For this review, take the finished solid that the model builds, in its own axes (mm). Face numbers are marked on the shaded views. A direction names the side the tool comes from. Coordinates: 2 decimals unless noted, no trailing zeros. Loops run counter-clockwise (first coordinate to the right, second up) from the corner with the lowest first, then second, coordinate; pieces in that order, holes last. Notation, with made-up numbers: (68, -8.5) -> (77, -8.5) arc R20 ccw to (77, 20.5) -> close; hole circle Ø2 at (80, 37.5). An arc over 180 degrees is marked (long way). Answer in a Markdown table with one row per item.
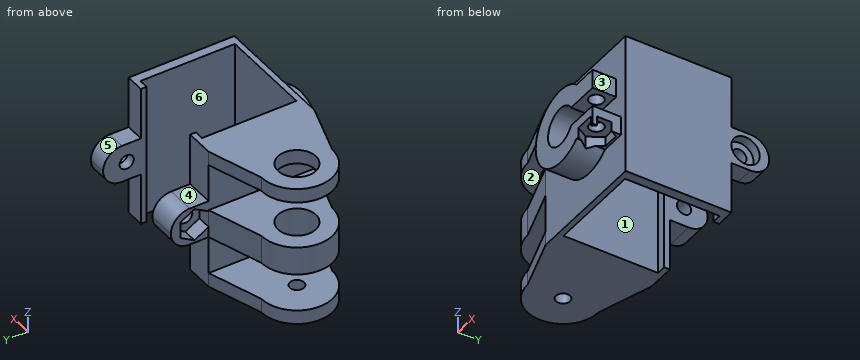
from build123d import *

# Parameters (mm, degrees)
F1_DEPTH  = 30
F3_DEPTH  = 6
F4_DEPTH  = 25
F6_DEPTH  = 15
F7_R      = 1.5
F8_DEPTH  = 25
F9_W      = 4
F9_H      = 8
F9_W_2    = 6
F10_DEPTH = 8
F11_R     = 3.99999
F12_R     = 1.5
F13_DEPTH = 25
F14_START = 27
F0_R      = 1.5
F14_DEPTH = 3
F15_START = 11
F15_DEPTH = 6
F16_DEPTH = 3
F17_R     = 4
F17_R_2   = 1.5
F18_DEPTH = 27
F12_R_2   = 3
F19_DEPTH = 2
F21_DEPTH = 3
F23_START = -2
F22_R     = 1.5
F23_DEPTH = 8


# Not quite as in the source:
# - a fillet or chamfer is up to 0.001 mm smaller than in the source, because OpenCascade refuses the exact size
# - a feature names something its author has since deleted; it is built from what else it names


with BuildPart() as f1:
    # F0 (on Top) → F1 (new body)
    with BuildSketch(Plane.XY):
        Polygon((20, 0), (0, 0), (0, 20), (2, 20), (2, 21.2), (-4, 21.2), (-4, -1.2), (22, -1.2), (22, 21.2), (18, 21.2), (18, 20), (20, 20), align=None)
    extrude(amount=F1_DEPTH)

    # F2 (on face) → F3 (join)
    with BuildSketch(Plane.XZ.offset(1.2)):
        with BuildLine():
            ThreePointArc((6, 15), (8.9647238196, 18.8637033052), (13.4641016151, 17))
            Line((13.4641016151, 17), (17.7459666924, 17))
            ThreePointArc((17.7459666924, 17), (16.8186436725, 19.1840289755), (15.2915026221, 21))
            ThreePointArc((15.2915026221, 21), (6.7084973779, 22.2915026221), (2, 15))
            Line((2, 15), (6, 15))
        make_face()
        with BuildLine():
            ThreePointArc((15.2915026221, 21), (16.8186436725, 19.1840289755), (17.7459666924, 17))
            Line((17.7459666924, 17), (20.4641016151, 17))
            Line((20.4641016151, 17), (20.4641016151, 21))
            Line((20.4641016151, 21), (15.2915026221, 21))
        make_face()
        with BuildLine():
            Line((20.4641016151, 13), (17.7459666924, 13))
            ThreePointArc((17.7459666924, 13), (16.8186436725, 10.8159710245), (15.2915026221, 9))
            Line((15.2915026221, 9), (20.4641016151, 9))
            Line((20.4641016151, 9), (20.4641016151, 13))
        make_face()
        with BuildLine():
            Line((17.7459666924, 13), (13.4641016151, 13))
            ThreePointArc((13.4641016151, 13), (8.9647238196, 11.1362966948), (6, 15))
            Line((6, 15), (2, 15))
            ThreePointArc((2, 15), (6.7084973779, 7.7084973779), (15.2915026221, 9))
            ThreePointArc((15.2915026221, 9), (16.8186436725, 10.8159710245), (17.7459666924, 13))
        make_face()
    extrude(amount=F3_DEPTH)

    # F2 (on face) → F4 (cut)
    with BuildSketch(Plane.XZ.offset(1.2)):
        with BuildLine():
            ThreePointArc((13.4641016151, 13), (13.8637033052, 13.9647238196), (14, 15))
            ThreePointArc((14, 15), (13.8637033052, 16.0352761804), (13.4641016151, 17))
            ThreePointArc((13.4641016151, 17), (8.9647238196, 18.8637033052), (6, 15))
            ThreePointArc((6, 15), (8.9647238196, 11.1362966948), (13.4641016151, 13))
        make_face()
    extrude(amount=-F4_DEPTH, mode=Mode.SUBTRACT)

    # F5 (on face) → F6 (cut)
    with BuildSketch(Plane.XY.offset(30)):
        Polygon((22, -1.2), (3, -1.2), (3, -2.2), (23, -2.2), (23, -1.2), align=None)
    extrude(amount=-F6_DEPTH, mode=Mode.SUBTRACT)

    # F7 (on face) → F8 (cut)
    with BuildSketch(Plane.XY.offset(21)):
        with Locations((17.8778021186, -4.7)):
            Circle(F7_R)
    extrude(amount=-F8_DEPTH, mode=Mode.SUBTRACT)

    # F9 (on face) → F10 (join)
    with BuildSketch(Plane(origin=(0, 21.2, 0), x_dir=(-1, 0, 0), z_dir=(0, 1, 0))):
        with Locations((-20, 15)):
            Rectangle(F9_W, F9_H)
        with Locations((1, 15)):
            Rectangle(F9_W_2, F9_H)
    extrude(amount=F10_DEPTH)

    # F11 (radius 4 in the source; OpenCascade refuses exactly that, so slightly less here)
    f11_edges = [f1.edges().sort_by_distance(p)[0] for p in [
        (20, 29.2, 19),
        (20, 29.2, 11),
        (-1, 29.2, 19),
        (-1, 29.2, 11),
    ]]
    fillet(f11_edges, radius=F11_R)

    # F12 (on face) → F13 (cut)
    with BuildSketch(Plane.YZ.offset(22)):
        with Locations((24.2, 15)):
            Circle(F12_R)
    extrude(amount=-F13_DEPTH, mode=Mode.SUBTRACT)

    # F0 (on Top) → F14 (join)
    with BuildSketch(Plane.XY.offset(F14_START)):
        with BuildLine():
            Line((-4, -1.2), (-4, 21.2))
            Line((-4, 21.2), (-15.5, 17.5))
            ThreePointArc((-15.5, 17.5), (-10.1966991411, 15.3033008589), (-8, 10))
            ThreePointArc((-8, 10), (-10.1966991411, 4.6966991411), (-15.5, 2.5))
            Line((-15.5, 2.5), (-4, -1.2))
        make_face()
        with BuildLine():
            ThreePointArc((-8, 10), (-10.1966991411, 15.3033008589), (-15.5, 17.5))
            ThreePointArc((-15.5, 17.5), (-23, 10), (-15.5, 2.5))
            ThreePointArc((-15.5, 2.5), (-10.1966991411, 4.6966991411), (-8, 10))
        make_face()
        with Locations((-15.5, 10)):
            Circle(F0_R, mode=Mode.SUBTRACT)
        Polygon((20, 0), (0, 0), (0, 20), (2, 20), (2, 21.2), (-4, 21.2), (-4, -1.2), (22, -1.2), (22, 21.2), (18, 21.2), (18, 20), (20, 20), align=None)
    extrude(amount=F14_DEPTH)

    # F0 (on Top) → F15 (join)
    with BuildSketch(Plane.XY.offset(F15_START)):
        with BuildLine():
            ThreePointArc((-8, 10), (-10.1966991411, 15.3033008589), (-15.5, 17.5))
            ThreePointArc((-15.5, 17.5), (-23, 10), (-15.5, 2.5))
            ThreePointArc((-15.5, 2.5), (-10.1966991411, 4.6966991411), (-8, 10))
        make_face()
        with Locations((-15.5, 10)):
            Circle(F0_R, mode=Mode.SUBTRACT)
        with BuildLine():
            Line((-4, -1.2), (-4, 21.2))
            Line((-4, 21.2), (-15.5, 17.5))
            ThreePointArc((-15.5, 17.5), (-10.1966991411, 15.3033008589), (-8, 10))
            ThreePointArc((-8, 10), (-10.1966991411, 4.6966991411), (-15.5, 2.5))
            Line((-15.5, 2.5), (-4, -1.2))
        make_face()
    extrude(amount=F15_DEPTH)

    # F0 (on Top) → F16 (join)
    with BuildSketch(Plane.XY):
        with BuildLine():
            ThreePointArc((-8, 10), (-10.1966991411, 15.3033008589), (-15.5, 17.5))
            ThreePointArc((-15.5, 17.5), (-23, 10), (-15.5, 2.5))
            ThreePointArc((-15.5, 2.5), (-10.1966991411, 4.6966991411), (-8, 10))
        make_face()
        with Locations((-15.5, 10)):
            Circle(F0_R, mode=Mode.SUBTRACT)
        with BuildLine():
            Line((-4, -1.2), (-4, 21.2))
            Line((-4, 21.2), (-15.5, 17.5))
            ThreePointArc((-15.5, 17.5), (-10.1966991411, 15.3033008589), (-8, 10))
            ThreePointArc((-8, 10), (-10.1966991411, 4.6966991411), (-15.5, 2.5))
            Line((-15.5, 2.5), (-4, -1.2))
        make_face()
    extrude(amount=F16_DEPTH)

    # F17 (on face) → F18 (cut)
    with BuildSketch(Plane.XY.offset(30)):
        with Locations((-15.5, 10)):
            Circle(F17_R)
        with Locations((-15.5, 10)):
            Circle(F17_R_2, mode=Mode.SUBTRACT)
    extrude(amount=-F18_DEPTH, mode=Mode.SUBTRACT)

    # F12 (on face) → F19 (cut)
    with BuildSketch(Plane.YZ.offset(22)):
        with Locations((24.2, 15)):
            Circle(F12_R_2)
        with Locations((24.2, 15)):
            Circle(F12_R, mode=Mode.SUBTRACT)
    extrude(amount=-F19_DEPTH, mode=Mode.SUBTRACT)

    # F20 (on face) → F21 (cut)
    with BuildSketch(Plane(origin=(-4, 0, 0), x_dir=(0, -1, 0), z_dir=(-1, 0, 0))):
        Polygon((-21.2, 13.2679491924), (-21.2, 16.7320508076), (-24.2, 18.4641016151), (-27.2, 16.7320508076), (-27.2, 13.2679491924), (-24.2, 11.5358983849), align=None)
    extrude(amount=-F21_DEPTH, mode=Mode.SUBTRACT)

    # F22 (on face) → F23 (cut)
    with BuildSketch(Plane.XY.offset(13).offset(F23_START)):
        Polygon((19.6098529262, -1.7), (16.1457513111, -1.7), (14.4137005035, -4.7), (15.8570761765, -7.2), (19.8985280608, -7.2), (20.4641016151, -6.2203978685), (20.4641016151, -3.1796021315), align=None)
        with Locations((17.8778021186, -4.7)):
            Circle(F22_R, mode=Mode.SUBTRACT)
    extrude(amount=-F23_DEPTH, mode=Mode.SUBTRACT)


solid = f1.part
Item 1: Take a section at B-B, the plane x = 10. State the section outline as (y, z) points, and give its area (3 significant figures).
Worked answers:
| item | result |
|---|---|
| outline | (-7.2, 7) -> (-1.2, 7) -> (-1.2, 0) -> (0, 0) -> (0, 11) -> (-7.2, 11) -> close; (-7.2, 19) -> (-2.2, 19) -> (-2.2, 23) -> (-7.2, 23) -> close; (-1.2, 19) -> (0, 19) -> (0, 30) -> (-1.2, 30) -> close |
| area | 70.4 mm² |
Item 2: For the marked faces 1, 2 and 3, list the 3-axis set-ups (+Z, -Z, +X, -X, +Y, -Y) from which the entire face can be reached by the end or side of a thin tool; tool diameter is ignored.
Worked answers:
| item | result |
|---|---|
| face 1 | +Z, -Z |
| face 2 | -X, +Y, -Y |
| face 3 | +Z, -Z, +X, -Y |
Item 3: The part is to be moulded in two halves that separate along Y. For the marked faces 4, 5 and 6, say which applies: +Y half, -Y half, draft (parallel to the pull), parting line (faces both ways), or undercut.
Worked answers:
| item | result |
|---|---|
| face 4 | draft |
| face 5 | +Y half |
| face 6 | undercut |
Item 4: Insertion check: pin 1 (1.2 mm diameter, centred on x = 21, y = 23, fed in from +Z); pin 2 (4 mm diameter, centred on y = 24.2, z = 15, fed in from +X); pin 3 (2 mm diameter, centred on y = -4, z = 11.5, fed in from +X); pin 4 (4.5 mm diameter, centred on x = 20, y = 22.5, fed in from -Z). Each pin has a flat end and moves straight along its axis. Give the tip position at first contact, or say it passes through.
Worked answers:
| item | result |
|---|---|
| pin 1 | z = 19 |
| pin 2 | x = 20 |
| pin 3 | x = 20.46 |
| pin 4 | z = 0 |
Item 5: Take a section at C-C, the plane x = -13. State the section outline as (y, z) points, and give its area (3 significant figures).
Worked answers:
| item | result |
|---|---|
| outline | (1.7, 0) -> (18.3, 0) -> (18.3, 3) -> (1.7, 3) -> close; (1.7, 11) -> (6.88, 11) -> (6.88, 17) -> (1.7, 17) -> close; (1.7, 27) -> (6.88, 27) -> (6.88, 30) -> (1.7, 30) -> close; (13.12, 11) -> (18.3, 11) -> (18.3, 17) -> (13.12, 17) -> close; (13.12, 27) -> (18.3, 27) -> (18.3, 30) -> (13.12, 30) -> close |
| area | 143 mm² |
Item 6: Take a section at A-A, the plane z = 24.5. State the section outline as (x, y) points.
Worked answers:
| item | result |
|---|---|
| outline | (-4, -1.2) -> (22, -1.2) -> (22, 21.2) -> (18, 21.2) -> (18, 20) -> (20, 20) -> (20, 0) -> (0, 0) -> (0, 20) -> (2, 20) -> (2, 21.2) -> (-4, 21.2) -> close |
Item 7: For L1, parallel to Z at x = -7, y = 0; L2, parallel to X at y = 11, z = 24.5; L3, parallel to Z at x = 20, y = -3.5, list the stretches that pass through material, from the lowest coordinate up.
Worked answers:
| item | result |
|---|---|
| L1 | 0 to 3, 11 to 17, 27 to 30 |
| L2 | -4 to 0, 20 to 22 |
| L3 | 11 to 13, 17 to 21 |
Item 8: Take a section at D-D, the plane x = 4. State the section outline as (y, z) points.
Worked answers:
| item | result |
|---|---|
| outline | (-7.2, 9.71) -> (-1.2, 9.71) -> (-1.2, 0) -> (0, 0) -> (0, 30) -> (-1.2, 30) -> (-1.2, 15) -> (-2.2, 15) -> (-2.2, 20.29) -> (-7.2, 20.29) -> close |
